Input: dimensioned drawing with shaded views. Units: mm. Origin: part minimum x, y, z. A direction names the side the tool comes from. Give positions to 0.01 mm unless a question says otherwise; leave off trailing zeros. Loops run counter-clockwise (first coordinate to the right, second up) from the corner with the lowest first, then second, coordinate; pieces in that order, holes last.
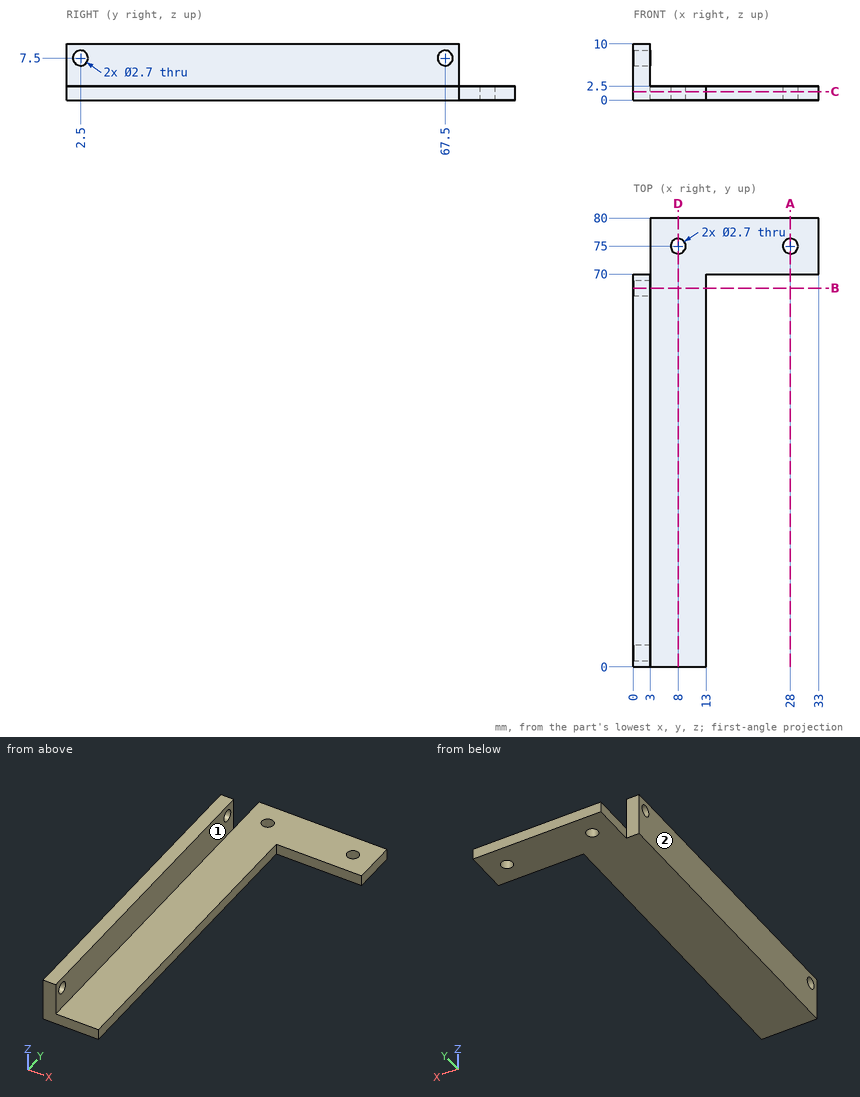
(1) Section B-B, the plane y = 67.5. Return the cut outline in (x, z).
A:
outline: (0, 0) - (13, 0) - (13, 2.5) - (3, 2.5) - (3, 6.15) - (0, 6.15) - close; (0, 8.85) - (3, 8.85) - (3, 10) - (0, 10) - close
(2) First-contact query: pin 1 (2 mm diameter, centred on x = 19, z = 1.5, fed in from -Y); pin 2 (4 mm diameter, centred on y = 26, z = 6, fed in from +X); pin 3 (1.6 mm diameter, centred on y = 2.5, z = 7.5, fed in from +X); pin 4 (0.8 mm diameter, centred on y = 73.5, z = 1.5, fed in from -X). Flat tips, straight axial feed; report the tip coordinate or a pass-through.
A:
pin 1: stops at y = 70
pin 2: stops at x = 3
pin 3: passes through
pin 4: stops at x = 3
(3) Section D-D, the plane x = 8. Return the cut outline in (y, z), then the cut area to 3 significant figures.
A:
outline: (0, 0) - (73.65, 0) - (73.65, 2.5) - (0, 2.5) - close; (76.35, 0) - (80, 0) - (80, 2.5) - (76.35, 2.5) - close
area: 193 mm2
(4) Section C-C, the plane z = 1.5. Return the cut outline in (x, y), then the cut area to 3 significant figures.
A:
outline: (0, 0) - (13, 0) - (13, 70) - (33, 70) - (33, 80) - (3, 80) - (3, 70) - (0, 70) - close; hole circle Ø2.7 at (8, 75); hole circle Ø2.7 at (28, 75)
area: 1,200 mm2
(5) Reachability of the marked faces 1 and 2 from +Z, -Z, +X, -X, +Y, -Y: full face, straight path, thin tool, end or side. Return the list, or none.
A:
face 1: +Z, +X, +Y, -Y
face 2: +Z, -Z, -X, +Y, -Y
(6) Ray query, line 1 along X through (y, z) = (75, 0.65); line 2 along Y through (x, z) = (8, 1.05); line 3 along X through (y, z) = (36, 9.5). Return the intervals inside material, ascending.
A:
line 1: x = 3 to 6.65, 9.35 to 26.65, 29.35 to 33
line 2: y = 0 to 73.65, 76.35 to 80
line 3: x = 0 to 3
(7) Section A-A, the plane x = 28. Return the cut outline in (y, z).
A:
outline: (70, 0) - (73.65, 0) - (73.65, 2.5) - (70, 2.5) - close; (76.35, 0) - (80, 0) - (80, 2.5) - (76.35, 2.5) - close
